The drawing under review shows one solid part. Ordinate dimensions are in mm from its lowest x, y, z. A direction names the side the tool comes from. Round coordinates to 2 decimals unless told otherwise and drop trailing zeros. Use a Markdown table: item, result. Add a question column.
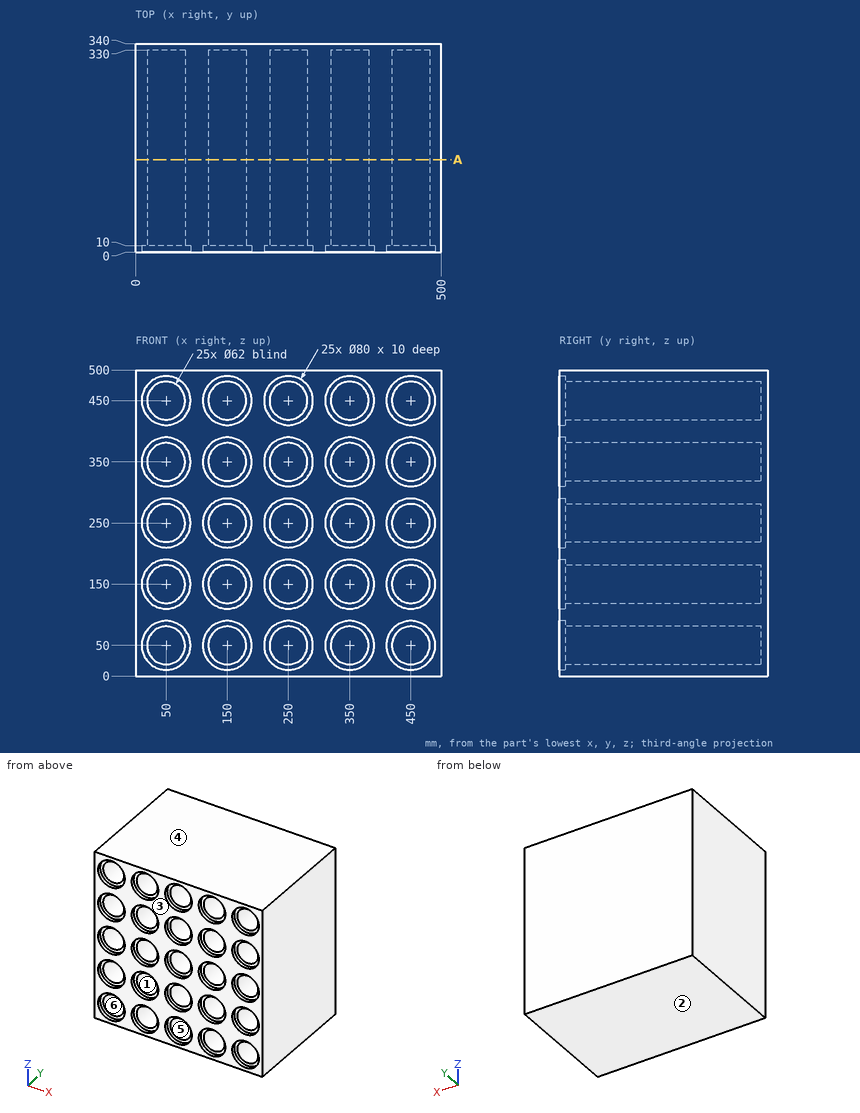
Q1. Draft analysis for pull direction Z (two halves, no side actions). For the marked faces 3, 4, 5 and 6, state which applies: released by +Z, released by -Z, zero draft, split by the parting line, or undercut.
Q2. Add section A-A, the plane y = 151. Give the number of separate pieces and of enclosed holes in the cut face, then the cut area to 3 significant figures.
Q3. For the marked faces 1 and 2, list the 3-axis set-ups (+Z, -Z, +X, -X, +Y, -Y) from which the entire face can be reached by the end or side of a thin tool; tool diameter is ignored.
Q4. To check wall thickness, follow line 1 along X through (y, z) = (138, 252); line 2 along X through (y, z) = (5, 150); line 3 along Z through (x, y) = (24, 298.5). State the ranges of each line that lie inside material, in increasing order.
Q5. For pin 1 (18.5 mm diameter, centred on x = 442.5, z = 238.5, fed in from -Y), flat-tipped, find the tip position at first contact; note if it passes through.
Return value:
| question | item | result |
|---|---|---|
| 1 | face 3 | zero draft |
| 1 | face 4 | released by +Z |
| 1 | face 5 | undercut |
| 1 | face 6 | undercut |
| 2 | separate pieces | 1 |
| 2 | enclosed holes | 25 |
| 2 | area | 175,000 mm² |
| 3 | face 1 | -Y |
| 3 | face 2 | -Z, +X, -X, +Y, -Y |
| 4 | line 1 | 0 to 19.06, 80.94 to 119.06, 180.94 to 219.06, 280.94 to 319.06, 380.94 to 419.06, 480.94 to 500 |
| 4 | line 2 | 0 to 10, 90 to 110, 190 to 210, 290 to 310, 390 to 410, 490 to 500 |
| 4 | line 3 | 0 to 33.12, 66.88 to 133.12, 166.88 to 233.12, 266.88 to 333.12, 366.88 to 433.12, 466.88 to 500 |
| 5 | pin 1 | y = 330 |
